Geometry check sheet. Reference: the model listing, model coordinates, mm. A direction names the side the tool comes from. Coordinates: 2 decimals unless noted, no trailing zeros. Order: outer loops, then holes, each group sorted by start corner. A loop starts at its lowest first (then second) coordinate and runs counter-clockwise, first axis right, second up. Notation, with made-up numbers: M 14,73 L 49,73 A22 cw 49,81 Z; hole C 20,32 d7. An arc over 180 degrees is marked long. One line per item, written item: value. Start each with the question number.
1) Thickness scan on L1, parallel to Y at x = -32, z = 2.5; L2, parallel to Z at x = 19, y = 27; L3, parallel to X at y = 26, z = 2. Record the ranges inside material, lowest first. Write a range as from..to.
2) Access from +Z, -Z, +X, -X, +Y, -Y to the whole of each face (thin tool, end or side, straight path). Record for faces 1 (the flat face through (-17, 6, 2)), 2 (the cylindrical face through (-30.188, 0.571, 1.972)), 3 (the flat face through (25.05, 7.44, 2.03)), 4 (the flat face through (-1, 4, 4)).
3) Sectioned sample at C-C, the plane z = 6.5. Enter the section's corners in (x, y), then the cut area to 3 significant figures.
4) Sectioned sample at B-B, the plane y = 0. Enter the section's corners in (x, z).
5) Draft check along Y on faces 5 (the flat face through (20, 4, 9)), 6 (the cylindrical face through (28.812, 0.571, 6.465)), 7 (the flat face through (9.171, 17.657, 1.972)). Enter one of: pulls with the +Y half, pulls with the -Y half, needs draft (parallel to the pull), parting line crosses it, or undercut.
6) Go/stop test with flat-tipped pins: P1, Ø5, axis at x = -3.5, z = 7.5, coming from the -Y side; P2, Ø1, axis at x = 8, y = 9, coming from the +Z side; P3, Ø5, axis at y = 12, z = 7.5, coming from the +X side; P4, Ø4.5, axis at x = -16, z = 1, coming from the +Y side. Record where each tip stops, or that it passes through.
7) Sectioned sample at A-A, the plane z = 2.75. Enter the section's corners in (x, y).
8) Sectioned sample at D-D, the plane x = 1.5. Enter the section's corners in (y, z), then the cut area to 3 significant figures.
```python
from build123d import *

# Parameters (mm, degrees)
F0_R     = 1.9
F1_DEPTH = 4
F2_R     = 1.9
F3_DEPTH = 5
F5_DEPTH = 4


with BuildPart() as f1:
    # F0 (on Top) → F1 (new body)
    with BuildSketch(Plane.XY):
        with BuildLine():
            Line((20.5060966544, 20.5060966544), (0, 0))
            Line((0, 0), (-26, 0))
            ThreePointArc((-26, 0), (-27.7573593129, -4.2426406871), (-32, -6))
            Line((-32, -6), (0, -6))
            ThreePointArc((0, -6), (2.2961005942, -5.5432771951), (4.2426406871, -4.2426406871))
            Line((4.2426406871, -4.2426406871), (28.9913780286, 20.5060966544))
            ThreePointArc((28.9913780286, 20.5060966544), (24.7487373415, 18.7487373415), (20.5060966544, 20.5060966544))
        make_face()
        with BuildLine():
            Line((-26, 0), (0, 0))
            Line((0, 0), (20.5060966544, 20.5060966544))
            ThreePointArc((20.5060966544, 20.5060966544), (18.7487373415, 24.7487373415), (20.5060966544, 28.9913780286))
            Line((20.5060966544, 28.9913780286), (-2.4852813742, 6))
            Line((-2.4852813742, 6), (-32, 6))
            ThreePointArc((-32, 6), (-27.7573593129, 4.2426406871), (-26, 0))
        make_face()
        with BuildLine():
            ThreePointArc((-32, -6), (-27.7573593129, -4.2426406871), (-26, 0))
            ThreePointArc((-26, 0), (-27.7573593129, 4.2426406871), (-32, 6))
            ThreePointArc((-32, 6), (-38, 0), (-32, -6))
        make_face()
        with Locations((-32, 0)):
            Circle(F0_R, mode=Mode.SUBTRACT)
        with BuildLine():
            ThreePointArc((20.5060966544, 28.9913780286), (18.7487373415, 24.7487373415), (20.5060966544, 20.5060966544))
            ThreePointArc((20.5060966544, 20.5060966544), (24.7487373415, 18.7487373415), (28.9913780286, 20.5060966544))
            ThreePointArc((28.9913780286, 20.5060966544), (30.2920145366, 22.4526367473), (30.7487373415, 24.7487373415))
            ThreePointArc((30.7487373415, 24.7487373415), (27.0448379357, 30.2920145366), (20.5060966544, 28.9913780286))
        make_face()
        with BuildLine():
            ThreePointArc((26.6487373415, 24.7487373415), (25.475835863, 22.9933662298), (23.4052344573, 23.4052344573))
            ThreePointArc((23.4052344573, 23.4052344573), (24.02163882, 26.5041084533), (26.6487373415, 24.7487373415))
        make_face(mode=Mode.SUBTRACT)
    extrude(amount=F1_DEPTH)

    # F2 (on face) → F3 (join)
    with BuildSketch(Plane.XY.offset(4)):
        with BuildLine():
            Line((28.9913780286, 20.5060966544), (4.2426406871, -4.2426406871))
            ThreePointArc((4.2426406871, -4.2426406871), (2.2961005942, -5.5432771951), (0, -6))
            Line((0, -6), (27, -6))
            ThreePointArc((27, -6), (31.6425330327, -3.8009060814), (32.8819440125, 1.1843709867))
            Line((32.8819440125, 1.1843709867), (28.9913780286, 20.5060966544))
        make_face()
        with Locations((27, 0)):
            Circle(F2_R, mode=Mode.SUBTRACT)
    extrude(amount=F3_DEPTH)

    # F4 (on face) → F5 (join)
    with BuildSketch(Plane(origin=(0, 0, 4), x_dir=(1, 0, 0), z_dir=(0, 0, -1))):
        with BuildLine():
            ThreePointArc((0, 6), (2.2961005942, 5.5432771951), (4.2426406871, 4.2426406871))
            Line((4.2426406871, 4.2426406871), (28.9913780286, -20.5060966544))
            Line((28.9913780286, -20.5060966544), (21, 6))
            Line((21, 6), (0, 6))
        make_face()
    extrude(amount=F5_DEPTH)


solid = f1.part
```
Final values:
1. L1: y = -6..-1.9, 1.9..6
1. L2: z = 0..4
1. L3: x = 17.51..23.32, 26.18..30.62
2. face 1: +Z, -Z, -X, +Y
2. face 2: +Z, -Z
2. face 3: -Z, +X, -Y
2. face 4: +Z, -X, +Y
3. outline: M 0,-6 L 27,-6 A6 ccw 32.88,1.18 L 28.99,20.51 L 4.24,-4.24 A6 cw Z; hole C 27,0 d3.8
3. area: 399 mm^2
4. outline: M -38,0 L -33.9,0 L -33.9,4 L -38,4 Z; M -30.1,0 L 22.81,0 L 22.81,4 L 25.1,4 L 25.1,9 L 8.49,9 L 8.49,4 L -30.1,4 Z; M 28.9,4 L 33,4 L 33,9 L 28.9,9 Z
5. face 5: needs draft
5. face 6: undercut
5. face 7: pulls with the +Y half
6. P1: passes through
6. P2: stops at z = 4
6. P3: stops at x = 31.21
6. P4: stops at y = 6
7. outline: M -32,-6 L 21,-6 L 28.99,20.51 A6 ccw 20.51,28.99 L -2.49,6 L -32,6 A6 ccw Z; hole C -32,0 d3.8; hole C 24.75,24.75 d3.8
8. outline: M -6,0 L 9.99,0 L 9.99,4 L -5.81,4 L -5.81,9 L -6,9 Z
8. area: 64.9 mm^2
